from build123d import *

# Parameters (mm, degrees)
ESBO_O1_W                                            = 315
ESBO_O1_H                                            = 100
RESSALTO_EXTRUS_O1_DEPTH                             = 19.02
ESBO_O2_R                                            = 2
CORTE_EXTRUS_O1_DEPTH                                = 25
ESBO_O4_R                                            = 5
CORTE_EXTRUS_O3_DEPTH                                = 20.02
ESBO_O5_R                                            = 3.3
CORTE_EXTRUS_O4_DEPTH                                = 90
REBAIXO_PARA_PARAFUSO_ALLEN_SEXTAVADO_DE_D           = 9
REBAIXO_PARA_PARAFUSO_ALLEN_SEXTAVADO_DE_DEPTH       = 19.02
REBAIXO_PARA_PARAFUSO_ALLEN_SEXTAVADO_DE_CBORE_D     = 15
REBAIXO_PARA_PARAFUSO_ALLEN_SEXTAVADO_DE_CBORE_DEPTH = 8.6
ESBO_O13_R                                           = 4
CORTE_EXTRUS_O8_DEPTH                                = 20
ESBO_O14_R                                           = 4
CORTE_EXTRUS_O9_DEPTH                                = 20
ESBO_O15_R                                           = 4
ESBO_O15_R_2                                         = 3
CORTE_EXTRUS_O10_DEPTH                               = 20.02
ESBO_O16_R                                           = 3.3
RESSALTO_EXTRUS_O2_DEPTH                             = 19.02
REBAIXO_PARA_PARAFUSO_ALLEN_SEXTAVAD_2_D             = 9
REBAIXO_PARA_PARAFUSO_ALLEN_SEXTAVAD_2_CBORE_D       = 15
REBAIXO_PARA_PARAFUSO_ALLEN_SEXTAVAD_2_CBORE_DEPTH   = 8.6


with BuildPart() as part:
    # Esboço1 → Ressalto-extrusão1 (new body)
    with BuildSketch(Plane(origin=(0, 0, 0), x_dir=(1, 0, 0), z_dir=(0, 1, 0))):
        Rectangle(ESBO_O1_W, ESBO_O1_H)
    extrude(amount=RESSALTO_EXTRUS_O1_DEPTH)

    # Esboço2 → Corte-extrusão1 (cut)
    with BuildSketch(Plane(origin=(0, 19.02, 0), x_dir=(1, 0, 0), z_dir=(0, 1, 0))):
        with Locations((143.5, 22.5)):
            Circle(ESBO_O2_R)
        with Locations((86.5, 22.5)):
            Circle(ESBO_O2_R)
        with Locations((86.5, -22.5)):
            Circle(ESBO_O2_R)
        with Locations((143.5, -22.5)):
            Circle(ESBO_O2_R)
        with Locations((-86.5, -22.45)):
            Circle(ESBO_O2_R)
        with Locations((-143.5, -22.45)):
            Circle(ESBO_O2_R)
        with Locations((-143.5, 22.55)):
            Circle(ESBO_O2_R)
        with Locations((-86.5, 22.55)):
            Circle(ESBO_O2_R)
    extrude(amount=-CORTE_EXTRUS_O1_DEPTH, mode=Mode.SUBTRACT)

    # Esboço4 → Corte-extrusão3 (cut, through all)
    with BuildSketch(Plane(origin=(0, 19.02, 0), x_dir=(1, 0, 0), z_dir=(0, 1, 0))):
        with Locations((-40, -32.999878702)):
            Circle(ESBO_O4_R)
        with Locations((-40, 33)):
            Circle(ESBO_O4_R)
        with Locations((40, 33)):
            Circle(ESBO_O4_R)
        with Locations((40, -33)):
            Circle(ESBO_O4_R)
    extrude(amount=-CORTE_EXTRUS_O3_DEPTH, mode=Mode.SUBTRACT)

    # Esboço5 → Corte-extrusão4 (cut)
    with BuildSketch(Plane(origin=(0, 19.02, 0), x_dir=(1, 0, 0), z_dir=(0, 1, 0))):
        Circle(ESBO_O5_R)
    extrude(amount=-CORTE_EXTRUS_O4_DEPTH, mode=Mode.SUBTRACT)

    # Rebaixo para parafuso Allen sextavado de
    with Locations(Plane(origin=(-143.5, 19.02, -22.55), x_dir=(0, 0, 1), z_dir=(0, 1, 0))):
        with Locations((0, 0), (45, 57), (0, 57), (45, 0), (0.05, 230), (0.05, 287), (45.05, 230), (45.05, 287)):
            CounterBoreHole(REBAIXO_PARA_PARAFUSO_ALLEN_SEXTAVADO_DE_D / 2, REBAIXO_PARA_PARAFUSO_ALLEN_SEXTAVADO_DE_CBORE_D / 2, REBAIXO_PARA_PARAFUSO_ALLEN_SEXTAVADO_DE_CBORE_DEPTH, depth=REBAIXO_PARA_PARAFUSO_ALLEN_SEXTAVADO_DE_DEPTH)

    # Esboço13 → Corte-extrusão8 (cut)
    with BuildSketch(Plane.XY.offset(50)):
        with Locations((-125, 9.51)):
            Circle(ESBO_O13_R)
        with Locations((-50, 9.51)):
            Circle(ESBO_O13_R)
        with Locations((50, 9.51)):
            Circle(ESBO_O13_R)
        with Locations((125, 9.51)):
            Circle(ESBO_O13_R)
    extrude(amount=-CORTE_EXTRUS_O8_DEPTH, mode=Mode.SUBTRACT)

    # Esboço14 → Corte-extrusão9 (cut)
    with BuildSketch(Plane(origin=(0, 0, -50), x_dir=(-1, 0, 0), z_dir=(0, 0, -1))):
        with Locations((-125, 9.51)):
            Circle(ESBO_O14_R)
        with Locations((-50, 9.51)):
            Circle(ESBO_O14_R)
        with Locations((50, 9.51)):
            Circle(ESBO_O14_R)
        with Locations((125, 9.51)):
            Circle(ESBO_O14_R)
    extrude(amount=-CORTE_EXTRUS_O9_DEPTH, mode=Mode.SUBTRACT)

    # Esboço15 → Corte-extrusão10 (cut, through all)
    with BuildSketch(Plane(origin=(0, 19.02, 0), x_dir=(1, 0, 0), z_dir=(0, 1, 0))):
        with Locations((30, 12.225)):
            Circle(ESBO_O15_R)
        with Locations((30, -12.225)):
            Circle(ESBO_O15_R)
        with Locations((-30, 12.225)):
            Circle(ESBO_O15_R)
        with Locations((-30, -12.225)):
            Circle(ESBO_O15_R)
        with Locations((-15, 0)):
            Circle(ESBO_O15_R_2)
        with Locations((15, 0)):
            Circle(ESBO_O15_R_2)
    extrude(amount=-CORTE_EXTRUS_O10_DEPTH, mode=Mode.SUBTRACT)

    # Esboço16 → Ressalto-extrusão2 (add)
    with BuildSketch(Plane(origin=(0, 19.02, 0), x_dir=(1, 0, 0), z_dir=(0, 1, 0))):
        Circle(ESBO_O16_R)
    extrude(amount=-RESSALTO_EXTRUS_O2_DEPTH)

    # Rebaixo para parafuso Allen sextavad 2 (through all)
    with Locations(Plane(origin=(-30, 19.02, -12.225), x_dir=(0, 0, 1), z_dir=(0, 1, 0))):
        with Locations((0, 0), (0, 60), (24.45, 60), (24.45, 0)):
            CounterBoreHole(REBAIXO_PARA_PARAFUSO_ALLEN_SEXTAVAD_2_D / 2, REBAIXO_PARA_PARAFUSO_ALLEN_SEXTAVAD_2_CBORE_D / 2, REBAIXO_PARA_PARAFUSO_ALLEN_SEXTAVAD_2_CBORE_DEPTH)


solid = part.part
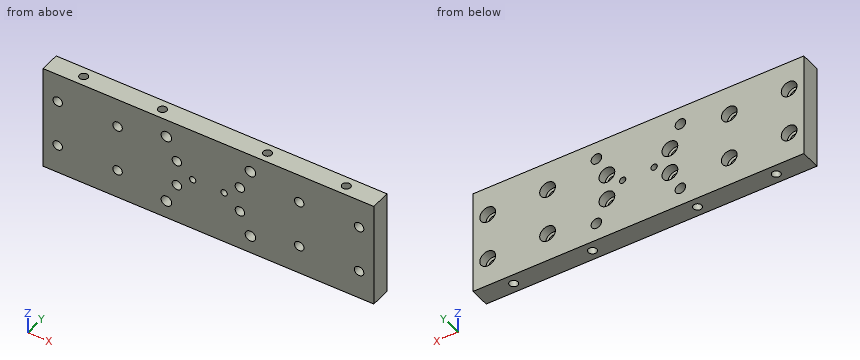
The listing builds one solid part. Answer for the finished solid, in the listing's coordinates (mm). Give positions to 0.01 mm unless a question says otherwise; leave off trailing zeros. Write each loop counter-clockwise with the first axis right and the second up, starting at its lowest first coordinate (ties: lowest second). Pieces come first, ordered by that corner, then holes.
Item 1: Find the intervals of material crossed by line 1 along X through (y, z) = (16.5, 22.5); line 2 along X through (y, z) = (5.25, 22.5); line 3 along Z through (x, y) = (87, 6.5), in increasing order.
Item 2: Section C-C, the plane x = -125 is taken. Write down the section's boundary in (y, z).
Item 3: Section B-B, the plane z = 0 is taken. Write down the section's boundary in (x, y).
Item 4: Section D-D, the plane z = 22.45 is taken. Count the separate pieces of the cut face and the enclosed holes in it, plus the area to 3 significant figures.
Item 5: Section A-A, the plane x = -86.5 is taken. Write down the section's boundary in (y, z), plus the area to 3 significant figures.
Item 6: Flat-ended cylindrical pins translate along their axes: P1, Ø7.5, axis at x = 27.5, z = 12, coming from the +Y side; P2, Ø2.5, axis at x = -127, y = 8, coming from the +Z side. Find the tip coordinate at first contact, or state that the pin passes through.
Completed:
1. line 1: x = -157.5 to -151, -136 to -94, -79 to 79, 94 to 136, 151 to 157.5
1. line 2: x = -157.5 to -148, -139 to -91, -82 to 82, 91 to 139, 148 to 157.5
1. line 3: z = -50 to -26.97, -18.03 to 18.03, 26.97 to 50
2. outline: (0, -50) - (5.51, -50) - (5.51, -30) - (13.51, -30) - (13.51, -50) - (19.02, -50) - (19.02, 50) - (13.51, 50) - (13.51, 30) - (5.51, 30) - (5.51, 50) - (0, 50) - close
3. outline: (-157.5, 0) - (-18, 0) - (-18, 19.02) - (-157.5, 19.02) - close; (-12, 0) - (12, 0) - (12, 19.02) - (-12, 19.02) - close; (18, 0) - (157.5, 0) - (157.5, 19.02) - (18, 19.02) - close
4. separate pieces: 5
4. enclosed holes: 0
4. area: 5,100 mm2
5. outline: (0, -50) - (19.02, -50) - (19.02, -30.05) - (10.42, -30.05) - (10.42, -27.05) - (0, -27.05) - close; (0, -18.05) - (10.42, -18.05) - (10.42, -15.05) - (19.02, -15.05) - (19.02, 14.95) - (10.42, 14.95) - (10.42, 17.95) - (0, 17.95) - close; (0, 26.95) - (10.42, 26.95) - (10.42, 29.95) - (19.02, 29.95) - (19.02, 50) - (0, 50) - close
5. area: 1,460 mm2
6. P1: stops at y = 10.42
6. P2: stops at z = 30
